```python
from build123d import *

# Parameters (mm, degrees)
SKETCH1_W           = 50
SKETCH1_H           = 220
SKETCH1_R           = 2
SKETCH1_R_2         = 2.5
SKETCH1_H_2         = 95
BOSS_EXTRUDE1_DEPTH = 3
BOSS_EXTRUDE2_START = 3
SKETCH1_4_W         = 220
SKETCH1_4_H         = 30
SKETCH1_4_R         = 2.25
BOSS_EXTRUDE2_DEPTH = 3


with BuildPart() as part:
    # Sketch1 → Boss-Extrude1 (new body)
    with BuildSketch(Plane(origin=(0, 0, 0), x_dir=(1, 0, 0), z_dir=(0, 1, 0))):
        with Locations((-85, 0)):
            Rectangle(SKETCH1_W, SKETCH1_H)
        with Locations(Location((-97, -69, 0), (0, 0, 270))):
            Circle(SKETCH1_R, mode=Mode.SUBTRACT)
        with Locations(Location((-73, -51, 0), (0, 0, 270))):
            Circle(SKETCH1_R, mode=Mode.SUBTRACT)
        with Locations(Location((-97, 69, 0), (0, 0, 270))):
            Circle(SKETCH1_R, mode=Mode.SUBTRACT)
        with Locations(Location((-73, 69, 0), (0, 0, 270))):
            Circle(SKETCH1_R, mode=Mode.SUBTRACT)
        with Locations(Location((-73, 51, 0), (0, 0, 270))):
            Circle(SKETCH1_R, mode=Mode.SUBTRACT)
        with Locations(Location((-97, 51, 0), (0, 0, 270))):
            Circle(SKETCH1_R, mode=Mode.SUBTRACT)
        with Locations(Location((-97, -51, 0), (0, 0, 270))):
            Circle(SKETCH1_R, mode=Mode.SUBTRACT)
        with Locations(Location((-73, -69, 0), (0, 0, 270))):
            Circle(SKETCH1_R, mode=Mode.SUBTRACT)
        with Locations(Location((-104.5, 104.5, 0), (0, 0, 270))):
            Circle(SKETCH1_R_2, mode=Mode.SUBTRACT)
        with Locations(Location((-104.5, -104.5, 0), (0, 0, 270))):
            Circle(SKETCH1_R_2, mode=Mode.SUBTRACT)
        with Locations((85, 0)):
            Rectangle(SKETCH1_W, SKETCH1_H)
        with Locations(Location((104.5, -104.5, 0), (0, 0, 270))):
            Circle(SKETCH1_R_2, mode=Mode.SUBTRACT)
        with Locations(Location((97, 69, 0), (0, 0, 270))):
            Circle(SKETCH1_R, mode=Mode.SUBTRACT)
        with Locations(Location((73, 51, 0), (0, 0, 270))):
            Circle(SKETCH1_R, mode=Mode.SUBTRACT)
        with Locations(Location((97, 51, 0), (0, 0, 270))):
            Circle(SKETCH1_R, mode=Mode.SUBTRACT)
        with Locations(Location((73, 69, 0), (0, 0, 270))):
            Circle(SKETCH1_R, mode=Mode.SUBTRACT)
        with Locations(Location((97, -69, 0), (0, 0, 270))):
            Circle(SKETCH1_R, mode=Mode.SUBTRACT)
        with Locations(Location((73, -69, 0), (0, 0, 270))):
            Circle(SKETCH1_R, mode=Mode.SUBTRACT)
        with Locations(Location((73, -51, 0), (0, 0, 270))):
            Circle(SKETCH1_R, mode=Mode.SUBTRACT)
        with Locations(Location((97, -51, 0), (0, 0, 270))):
            Circle(SKETCH1_R, mode=Mode.SUBTRACT)
        with Locations(Location((104.5, 104.5, 0), (0, 0, 270))):
            Circle(SKETCH1_R_2, mode=Mode.SUBTRACT)
        with Locations((-85, -62.5)):
            Rectangle(SKETCH1_W, SKETCH1_H_2)
        with Locations(Location((-104.5, -104.5, 0), (0, 0, 270))):
            Circle(SKETCH1_R_2, mode=Mode.SUBTRACT)
        with Locations(Location((-97, -69, 0), (0, 0, 270))):
            Circle(SKETCH1_R, mode=Mode.SUBTRACT)
        with Locations(Location((-73, -69, 0), (0, 0, 270))):
            Circle(SKETCH1_R, mode=Mode.SUBTRACT)
        with Locations(Location((-97, -51, 0), (0, 0, 270))):
            Circle(SKETCH1_R, mode=Mode.SUBTRACT)
        with Locations(Location((-73, -51, 0), (0, 0, 270))):
            Circle(SKETCH1_R, mode=Mode.SUBTRACT)
        with Locations((-85, 62.5)):
            Rectangle(SKETCH1_W, SKETCH1_H_2)
        with Locations(Location((-97, 51, 0), (0, 0, 270))):
            Circle(SKETCH1_R, mode=Mode.SUBTRACT)
        with Locations(Location((-73, 51, 0), (0, 0, 270))):
            Circle(SKETCH1_R, mode=Mode.SUBTRACT)
        with Locations(Location((-97, 69, 0), (0, 0, 270))):
            Circle(SKETCH1_R, mode=Mode.SUBTRACT)
        with Locations(Location((-73, 69, 0), (0, 0, 270))):
            Circle(SKETCH1_R, mode=Mode.SUBTRACT)
        with Locations(Location((-104.5, 104.5, 0), (0, 0, 270))):
            Circle(SKETCH1_R_2, mode=Mode.SUBTRACT)
        with Locations((85, 62.5)):
            Rectangle(SKETCH1_W, SKETCH1_H_2)
        with Locations(Location((73, 51, 0), (0, 0, 270))):
            Circle(SKETCH1_R, mode=Mode.SUBTRACT)
        with Locations(Location((97, 51, 0), (0, 0, 270))):
            Circle(SKETCH1_R, mode=Mode.SUBTRACT)
        with Locations(Location((73, 69, 0), (0, 0, 270))):
            Circle(SKETCH1_R, mode=Mode.SUBTRACT)
        with Locations(Location((97, 69, 0), (0, 0, 270))):
            Circle(SKETCH1_R, mode=Mode.SUBTRACT)
        with Locations(Location((104.5, 104.5, 0), (0, 0, 270))):
            Circle(SKETCH1_R_2, mode=Mode.SUBTRACT)
        with Locations((85, -62.5)):
            Rectangle(SKETCH1_W, SKETCH1_H_2)
        with Locations(Location((104.5, -104.5, 0), (0, 0, 270))):
            Circle(SKETCH1_R_2, mode=Mode.SUBTRACT)
        with Locations(Location((73, -69, 0), (0, 0, 270))):
            Circle(SKETCH1_R, mode=Mode.SUBTRACT)
        with Locations(Location((97, -69, 0), (0, 0, 270))):
            Circle(SKETCH1_R, mode=Mode.SUBTRACT)
        with Locations(Location((73, -51, 0), (0, 0, 270))):
            Circle(SKETCH1_R, mode=Mode.SUBTRACT)
        with Locations(Location((97, -51, 0), (0, 0, 270))):
            Circle(SKETCH1_R, mode=Mode.SUBTRACT)
    extrude(amount=BOSS_EXTRUDE1_DEPTH)

    # Sketch1<4> → Boss-Extrude2 (add)
    with BuildSketch(Plane(origin=(0, 0, 0), x_dir=(1, 0, 0), z_dir=(0, 1, 0)).offset(BOSS_EXTRUDE2_START)):
        Rectangle(SKETCH1_4_W, SKETCH1_4_H)
        with Locations(Location((6.575, 9, 0), (0, 0, 270))):
            Circle(SKETCH1_4_R, mode=Mode.SUBTRACT)
        with Locations(Location((-6.575, -9, 0), (0, 0, 270))):
            Circle(SKETCH1_4_R, mode=Mode.SUBTRACT)
        with Locations(Location((6.575, -9, 0), (0, 0, 270))):
            Circle(SKETCH1_4_R, mode=Mode.SUBTRACT)
        with Locations(Location((-6.575, 9, 0), (0, 0, 270))):
            Circle(SKETCH1_4_R, mode=Mode.SUBTRACT)
    extrude(amount=BOSS_EXTRUDE2_DEPTH)


solid = part.part
```
Can you work these out from the model? Positions are in its coordinate system, mm. A direction names the side the tool comes from. Give positions to 0.01 mm unless a question says otherwise; leave off trailing zeros. Loops run counter-clockwise (first coordinate to the right, second up) from the corner with the lowest first, then second, coordinate; pieces in that order, holes last. Notation, with made-up numbers: M 80.25,41.25 L 137.25,41.25 A25 ccw 137.25,66.25 Z; hole C -11.5,55 d7. An arc over 180 degrees is marked long. One line per question, with ' | ' between items. Start each with the question number.
Q1. If we section it at B-B (y = 2.05): State how many separate pieces and enclosed holes the cut face has, plus the area to 3 significant figures.
Q2. If we mould it in two halves opening along X, with no side actions, what happens to faces 4 (the cylindrical face through (-103.749, 1.479, 106.885)), 5 (the flat face through (-110, 2, 2)), 6 (the flat face through (85, 3, -63)), 7 (the flat face through (110, 2, 2))? For each: +X half, -X half, draft (parallel to the pull), parting line (faces both ways), or undercut.
Q3. For pin 1 Ø1.5 at (x, y) = (-1.5, 4.5) entering from -Z; pin 2 Ø6.5 at (x, z) = (-97, 69) entering from +Y; pin 3 Ø3.5 at (x, z) = (97, -51) entering from -Y; pin 4 Ø7 at (x, z) = (6.575, 9) entering from -Y, each with a flat end and sliding along its axis, tell me the tip position at first contact or that it passes through.
Q4. If we section it at C-C (x = 104.5): Please give me the cut outline in (y, z), plus the area to 3 significant figures.
Q5. If we section it at D-D (z = 104.5): Please give me the cut outline in (x, y), plus the area to 3 significant figures.
Q6. For faces 1 (the flat face through (-1, 3, 0)), 2 (the flat face through (85, 3, 62)), 3 (the flat face through (-85, 3, -63)), which set-ups out of +Z, -Z, +X, -X, +Y, -Y let a thin tool reach every point of the face, with its end or its side?
Q7. If I drill on line 1 (X direction, y = 2, z = 51); line 2 (X direction, y = 1.7, z = 104.5); line 3 (X direction, y = 1.05, z = -47), over which ranges is the centre line in solid material (lowest first)? Write a range as from..to.
Q8. If we section it at A-A (z = 37.5): Please give me the cut outline in (x, y).
Computed:
1) separate pieces: 2 | enclosed holes: 20 | area: 21,700 mm²
2) face 4: undercut | face 5: -X half | face 6: draft | face 7: +X half
3) pin 1: stops at z = -15 | pin 2: stops at y = 3 | pin 3: passes through | pin 4: stops at y = 3
4) outline: M 0,-110 L 3,-110 L 3,-107 L 0,-107 Z; M 0,-102 L 3,-102 L 3,-15 L 6,-15 L 6,15 L 3,15 L 3,102 L 0,102 Z; M 0,107 L 3,107 L 3,110 L 0,110 Z | area: 720 mm²
5) outline: M -110,0 L -107,0 L -107,3 L -110,3 Z; M -102,0 L -60,0 L -60,3 L -102,3 Z; M 60,0 L 102,0 L 102,3 L 60,3 Z; M 107,0 L 110,0 L 110,3 L 107,3 Z | area: 270 mm²
6) face 1: +Z, -Z, -Y | face 2: +Z, +X, -X, +Y | face 3: -Z, +X, -X, +Y
7) line 1: x = -110..-99, -95..-75, -71..-60, 60..71, 75..95, 99..110 | line 2: x = -110..-107, -102..-60, 60..102, 107..110 | line 3: x = -110..-60, 60..110
8) outline: M -110,0 L -60,0 L -60,3 L -110,3 Z; M 60,0 L 110,0 L 110,3 L 60,3 Z
